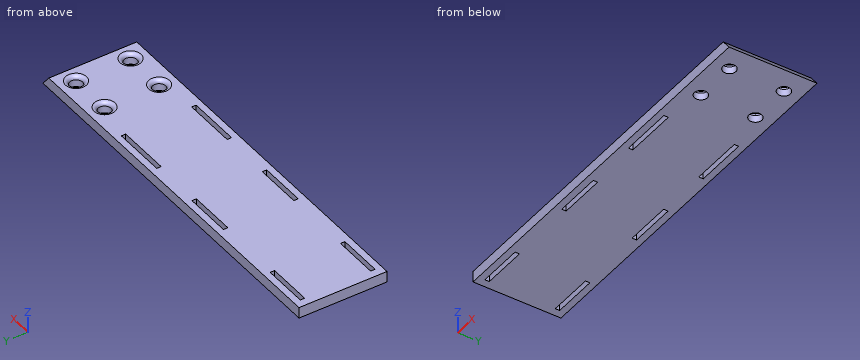
from build123d import *

# Parameters (mm, degrees)
F0_W     = 50.8
F0_H     = 215.9
F0_R     = 3.7465
F0_W_2   = 2.54
F0_H_2   = 30.5881015956
F0_R_2   = 3.7211
F0_H_3   = 27.157658129
F0_H_4   = 26.0141715407
F1_DEPTH = 6.35
F2_ANGLE = 180
F4_DEPTH = 50.8
F5_ANGLE = 90
F6_ANGLE = -90
F7_R     = 2.286


with BuildPart() as f1:
    # F0 (on Front) → F1 (new body)
    with BuildSketch(Plane.XZ):
        with Locations((-10.9999279406, -8.0348854876)):
            Rectangle(F0_W, F0_H)
        with Locations((-26.7352279406, -106.9043854876)):
            Circle(F0_R, mode=Mode.SUBTRACT)
        with Locations((-26.7352279406, -82.2409854876)):
            Circle(F0_R, mode=Mode.SUBTRACT)
        with Locations((-31.3199279406, -43.8153201211)):
            Rectangle(F0_W_2, F0_H_2, mode=Mode.SUBTRACT)
        with Locations((4.7353720594, -106.9043854876)):
            Circle(F0_R, mode=Mode.SUBTRACT)
        with Locations((4.7607720594, -82.2663985804)):
            Circle(F0_R_2, mode=Mode.SUBTRACT)
        with Locations((9.3200720594, -43.8153201211)):
            Rectangle(F0_W_2, F0_H_2, mode=Mode.SUBTRACT)
        with Locations((-31.3199279406, 15.4236085401)):
            Rectangle(F0_W_2, F0_H_3, mode=Mode.SUBTRACT)
        with Locations((-31.3199279406, 82.3172128331)):
            Rectangle(F0_W_2, F0_H_4, mode=Mode.SUBTRACT)
        with Locations((9.3200720594, 15.4236085401)):
            Rectangle(F0_W_2, F0_H_3, mode=Mode.SUBTRACT)
        with Locations((9.3200720594, 82.3172128331)):
            Rectangle(F0_W_2, F0_H_4, mode=Mode.SUBTRACT)
    extrude(amount=F1_DEPTH)


with BuildPart() as f1_1:
    # F2: moved
    add(f1.part.rotate(Axis((-10.9999279406, 0, 99.9151145124), (1, 0, 0)), F2_ANGLE))

    # F3 (on face) → F4 (join)
    with BuildSketch(Plane.YZ.offset(14.4000720594)):
        Polygon((0, 320.8044469357), (0, 315.8151145124), (6.35, 315.8151145124), align=None)
    extrude(amount=-F4_DEPTH)


with BuildPart() as f1_2:
    # F5: moved
    add(f1_1.part.rotate(Axis((-10.9999279406, 0, 99.9151145124), (1, 0, 0)), F5_ANGLE))


with BuildPart() as f1_3:
    # F6: moved
    add(f1_2.part.rotate(Axis((14.4000720594, 0, 103.0901145124), (0, 0, -1)), F6_ANGLE))

    # F7
    f7_edges = [f1_3.edges().sort_by_distance(p)[0] for p in [
        (196.581585, -13.3604, 106.265115),
        (221.219572, -13.4112, 106.265115),
        (196.556172, -44.8818, 106.265115),
        (221.219572, -44.8818, 106.265115),
    ]]
    fillet(f7_edges, radius=F7_R)


solid = f1_3.part
Can you work these out from the model? Positions are in its coordinate system, mm. Round coordinates to 2 decimals unless told otherwise and drop trailing zeros. Loops run counter-clockwise (first coordinate to the right, second up) from the corner with the lowest first, then second, coordinate; pieces in that order, holes last. Notation, with made-up numbers: (73.5, -21.75) - (113.5, -21.75) arc R20 ccw to (113.5, 12.25) - close; hole circle Ø6 at (80, 87). An arc over 180 degrees is marked (long way). Use CSV: the item, a comma, the result in double quotes. Start each with the question number.
1) If we section it at B-B on z = 105: Count the separate pieces of the cut face and the enclosed holes in it, plus the area to 3 significant figures.
2) Please list where these lines run through material, in increasing order: probe 1 along Y at (x, z) = (103.5, 102); probe 2 along X at (y, z) = (-4.5, 101.75). Write a range as [from, to].
3) If we section it at A-A on x = 42: Write out the boundary of the cut face in (y, z).
4) For pin 1 Ø12 at (x, y) = (221.22, -41.14) entering from -Z; pin 2 Ø6 at (x, y) = (221.22, -9.66) entering from -Z; pin 3 Ø0.8 at (y, z) = (-4.5, 104.5) entering from +X; pin 4 Ø1.5 at (y, z) = (-29, 100.5) entering from +X, each with a flat end and sliding along its axis, tell me the tip position at first contact or that it passes through.
Geometry results:
1,separate pieces,"1"
1,enclosed holes,"10"
1,area,"10,400 mm2"
2,probe 1,"y = [-50.8, -46.99], [-44.45, -6.35], [-3.81, 0]"
2,probe 2,"x = [14.4, 18.99], [45.01, 85.31], [112.47, 142.84], [173.42, 233.85]"
3,outline,"(-50.8, 99.92) - (-46.99, 99.92) - (-46.99, 106.27) - (-50.8, 106.27) - close; (-44.45, 99.92) - (-6.35, 99.92) - (-6.35, 106.27) - (-44.45, 106.27) - close; (-3.81, 99.92) - (0, 99.92) - (0, 106.27) - (-3.81, 106.27) - close"
4,pin 1,"stops at z = 99.92"
4,pin 2,"passes through"
4,pin 3,"stops at x = 232"
4,pin 4,"stops at x = 235.29"
